```python
from build123d import *

# Parameters (mm, degrees)
SKETCH_1_R      = 15
EXTRUDE_1_DEPTH = 70
SKETCH_2_R      = 27.5
EXTRUDE_2_DEPTH = 95
CHAMFER_1_SIZE  = 1
SKETCH_3_W      = 5.21377611
SKETCH_3_H      = 1.5


with BuildPart() as part:
    # 草图1 → 凸台-拉伸1 (new body)
    with BuildSketch(Plane.XY):
        Circle(SKETCH_1_R)
    extrude(amount=EXTRUDE_1_DEPTH)

    # 草图2 → 凸台-拉伸2 (add)
    with BuildSketch(Plane.XY.offset(70)):
        Circle(SKETCH_2_R)
    extrude(amount=EXTRUDE_2_DEPTH)

    # 倒角1
    chamfer_1_edges = [part.edges().sort_by_distance(p)[0] for p in [
        (-15, 0, 0),
        (-27.5, 0, 70),
        (-27.5, 0, 165),
    ]]
    chamfer(chamfer_1_edges, length=CHAMFER_1_SIZE)

    # 草图3 → 切除-旋转1 (revolve, cut)
    with BuildSketch(Plane(origin=(0, 0, 0), x_dir=(1, 0, 0), z_dir=(0, 1, 0)), mode=Mode.PRIVATE) as cut_revolve_1_sk:
        with Locations((16.606888055, -58.25)):
            Rectangle(SKETCH_3_W, SKETCH_3_H)
        with Locations((16.606888055, -4.25)):
            Rectangle(SKETCH_3_W, SKETCH_3_H)
    revolve(cut_revolve_1_sk.sketch.rotate(Axis((0, 0, -18.215048165), (0, 0, 1)), 180), axis=Axis((0, 0, -18.215048165), (0, 0, 1)), mode=Mode.SUBTRACT)


solid = part.part
```
CAD build for the part. Positions are in the model's coordinates, mm. A direction names the side the tool comes from. Coordinates: 2 decimals unless noted, no trailing zeros. Order: outer loops, then holes, each group sorted by start corner. A loop starts at its lowest first (then second) coordinate and runs counter-clockwise, first axis right, second up.
(1) Mould opens along Z. For faces 4 (the face through (0, 0, 165)), 5 (the face through (-14.985, 0.66, 64.423)), 6 (the face through (-13.35, -4.21, 4.24)), 7 (the face through (0, 0, 0)) say: released by +Z, released by -Z, zero draft, split by the parting line, or undercut.
Solution:
face 4: released by +Z
face 5: zero draft
face 6: undercut
face 7: released by -Z
(2) Saw through at C-C, the plane z = 42. Write the cut outline in (x, y), and give its area (3 significant figures).
Solution:
outline: circle Ø30 at (0, 0)
area: 707 mm2
(3) Drill centre lines: L1, parallel to Z at x = -13.5, y = 4.5; L2, parallel to Y at x = 0.5, z = 66; L3, parallel to Z at x = -16, y = 7. Where is each one in solid material? Low to high.
Solution:
L1: z = 0.23 to 3.5, 5 to 57.5, 59 to 165
L2: y = -14.99 to 14.99
L3: z = 70 to 165
(4) Which spindle directions (+Z, -Z, +X, -X, +Y, -Y) get a long thin tool onto all of the face, cutting with end or side? Do faces 1 (the face through (-14.985, 0.66, 30.882)), 2 (the face through (-5.961, -26.846, 116.849)), 3 (the face through (-13.35, -4.21, 58.24)). Say none if no direction does.
Solution:
face 1: -Z
face 2: +Z, -Z
face 3: none
(5) Pin check, flat tips, straight feed: pin 1 Ø16 at (x, y) = (-5, -10) entering from -Z; pin 2 Ø8 at (y, z) = (-11, 31) entering from -X; pin 3 Ø1 at (x, z) = (8.5, 24.5) entering from +Y; pin 4 Ø12 at (y, z) = (-7, 25.5) entering from -X. Stop position of each tip, or through.
Solution:
pin 1: stops at z = 0
pin 2: stops at x = -13.27
pin 3: stops at y = 12.69
pin 4: stops at x = -14.97
(6) Saw through at D-D, the plane z = 124. Write the cut outline in (x, y).
Solution:
outline: circle Ø55 at (0, 0)
